Verification items for the finished model (mm, model axes). Face numbers are marked on the shaded views. A direction names the side the tool comes from. Round coordinates to 2 decimals unless told otherwise and drop trailing zeros. Loops run counter-clockwise (first coordinate to the right, second up) from the corner with the lowest first, then second, coordinate; pieces in that order, holes last. Notation, with made-up numbers: M 37,86 L 44,86 A32 cw 44,114 Z; hole C 9.25,-25.5 d10. An arc over 180 degrees is marked long. One line per item, written item: value.
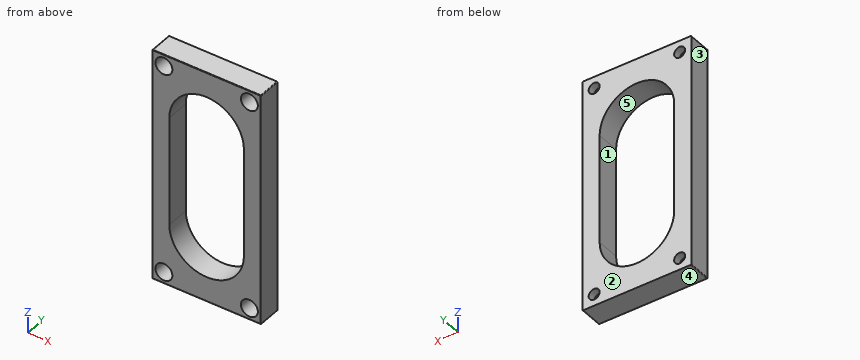
from build123d import *

# Parameters (mm, degrees)
F0_W      = 44.45
F0_H      = 95.25
F0_R      = 3.4671
F1_DEPTH  = 6.35
F0_R_2    = 2.2479
F1_FACE_W = 44.45
F1_FACE_H = 95.25
F1_FACE_R = 3.4671
F2_DEPTH  = 3.175
F3_R      = 0.254


# Not quite as in the source:
# - a feature names something its author has since deleted; it is built from what else it names


with BuildPart() as f1:
    # F0 (on Front) → F1 (new body)
    with BuildSketch(Plane.XZ):
        Rectangle(F0_W, F0_H)
        with Locations((-17.4625, -42.8625)):
            Circle(F0_R, mode=Mode.SUBTRACT)
        with Locations((17.4625, -42.8625)):
            Circle(F0_R, mode=Mode.SUBTRACT)
        with Locations((-17.4625, 42.8625)):
            Circle(F0_R, mode=Mode.SUBTRACT)
        with BuildLine():
            ThreePointArc((-15.24, 22.225), (0, 37.465), (15.24, 22.225))
            Line((15.24, 22.225), (15.24, -22.225))
            ThreePointArc((15.24, -22.225), (0, -37.465), (-15.24, -22.225))
            Line((-15.24, -22.225), (-15.24, 22.225))
        make_face(mode=Mode.SUBTRACT)
        with Locations((17.4625, 42.8625)):
            Circle(F0_R, mode=Mode.SUBTRACT)
    extrude(amount=F1_DEPTH)

    # F0 (on Front) + F1_face (on face) → F2 (join)
    with BuildSketch(Plane.XZ):
        Rectangle(F0_W, F0_H)
        with Locations((-17.4625, -42.8625)):
            Circle(F0_R, mode=Mode.SUBTRACT)
        with Locations((17.4625, -42.8625)):
            Circle(F0_R, mode=Mode.SUBTRACT)
        with Locations((-17.4625, 42.8625)):
            Circle(F0_R, mode=Mode.SUBTRACT)
        with BuildLine():
            ThreePointArc((-15.24, 22.225), (0, 37.465), (15.24, 22.225))
            Line((15.24, 22.225), (15.24, -22.225))
            ThreePointArc((15.24, -22.225), (0, -37.465), (-15.24, -22.225))
            Line((-15.24, -22.225), (-15.24, 22.225))
        make_face(mode=Mode.SUBTRACT)
        with Locations((17.4625, 42.8625)):
            Circle(F0_R, mode=Mode.SUBTRACT)
        with Locations((-17.4625, 42.8625)):
            Circle(F0_R)
        with Locations((-17.4625, 42.8625)):
            Circle(F0_R_2, mode=Mode.SUBTRACT)
        with Locations((17.4625, 42.8625)):
            Circle(F0_R)
        with Locations((17.4625, 42.8625)):
            Circle(F0_R_2, mode=Mode.SUBTRACT)
        with Locations((-17.4625, -42.8625)):
            Circle(F0_R)
        with Locations((-17.4625, -42.8625)):
            Circle(F0_R_2, mode=Mode.SUBTRACT)
        with Locations((17.4625, -42.8625)):
            Circle(F0_R)
        with Locations((17.4625, -42.8625)):
            Circle(F0_R_2, mode=Mode.SUBTRACT)
    with BuildSketch(Plane.XZ.offset(6.35)):
        Rectangle(F1_FACE_W, F1_FACE_H)
        with Locations((-17.4625, -42.8625)):
            Circle(F1_FACE_R, mode=Mode.SUBTRACT)
        with Locations((17.4625, -42.8625)):
            Circle(F1_FACE_R, mode=Mode.SUBTRACT)
        with Locations((-17.4625, 42.8625)):
            Circle(F1_FACE_R, mode=Mode.SUBTRACT)
        with BuildLine():
            Line((-15.24, -22.225), (-15.24, 22.225))
            ThreePointArc((-15.24, 22.225), (0, 37.465), (15.24, 22.225))
            Line((15.24, 22.225), (15.24, -22.225))
            ThreePointArc((15.24, -22.225), (0, -37.465), (-15.24, -22.225))
        make_face(mode=Mode.SUBTRACT)
        with Locations((17.4625, 42.8625)):
            Circle(F1_FACE_R, mode=Mode.SUBTRACT)
    extrude(amount=F2_DEPTH)

    # F3
    f3_edges = [f1.edges().sort_by_distance(p)[0] for p in [
        (-22.225, -9.525, 0),
        (0, -9.525, -47.625),
        (22.225, -9.525, 0),
        (0, -9.525, 47.625),
        (-22.225, -4.7625, 47.625),
        (22.225, -4.7625, 47.625),
        (22.225, -4.7625, -47.625),
        (-22.225, -4.7625, -47.625),
    ]]
    fillet(f3_edges, radius=F3_R)


solid = f1.part
(1) Depth check by flat-ended pin: pin 1 Ø9 at (x, z) = (17.46, -42.86) entering from +Y; pin 2 Ø3.5 at (x, z) = (17, -42) entering from -Y (3 decimals); pin 3 Ø4 at (x, z) = (17.46, -42.86) entering from -Y. Enter the tip coordinate at first touch or a pass-through.
Completed:
pin 1: stops at y = 0
pin 2: stops at y = -3.175
pin 3: passes through
(2) Sectioned sample at C-C on y = -1.75. Count the separate pieces of the cut face and the enclosed holes in it, and give its area (3 significant figures).
Completed:
separate pieces: 1
enclosed holes: 5
area: 2,090 mm^2
(3) Tool access check on the marked faces 1 and 2. Record the directions out of +Z, -Z, +X, -X, +Y, -Y that give a thin tool (end or side, any length) a straight path to the whole face; none if there is none.
Completed:
face 1: +Y, -Y
face 2: +Z, -Z, +X, -X, +Y
(4) Sectioned sample at B-B on z = -9. Enter the section's corners in (x, y) (3 decimals).
Completed:
outline: M -22.225,-9.271 A0.254 ccw -21.971,-9.525 L -15.24,-9.525 L -15.24,0 L -22.225,0 Z; M 15.24,-9.525 L 21.971,-9.525 A0.254 ccw 22.225,-9.271 L 22.225,0 L 15.24,0 Z
(5) Sectioned sample at A-A on x = 0. Enter the section's corners in (y, z) (3 decimals), and give its area (3 significant figures).
Completed:
outline: M -9.525,-47.371 A0.254 ccw -9.271,-47.625 L 0,-47.625 L 0,-37.465 L -9.525,-37.465 Z; M -9.525,37.465 L 0,37.465 L 0,47.625 L -9.271,47.625 A0.254 ccw -9.525,47.371 Z
area: 194 mm^2
(6) Sectioned sample at D-D on z = -42. Enter the section's corners in (x, y) (3 decimals), and give its area (3 significant figures).
Completed:
outline: M -22.225,-9.271 A0.254 ccw -21.971,-9.525 L -20.821,-9.525 L -20.821,-3.175 L -19.538,-3.175 L -19.538,0 L -22.225,0 Z; M -15.387,-3.175 L -14.104,-3.175 L -14.104,-9.525 L 14.104,-9.525 L 14.104,-3.175 L 15.387,-3.175 L 15.387,0 L -15.387,0 Z; M 19.538,-3.175 L 20.821,-3.175 L 20.821,-9.525 L 21.971,-9.525 A0.254 ccw 22.225,-9.271 L 22.225,0 L 19.538,0 Z
area: 312 mm^2
(7) Mould release check, pull along X, two halves, no side actions. Record for the marked faces 3, 4 and 5: +X half, -X half, draft (parallel to the pull), parting line (faces both ways), or undercut.
Completed:
face 3: -X half
face 4: draft
face 5: undercut
(8) Thickness scan on L1, parallel to Z at x = -17.5, y = -1.25 (3 decimals); L2, parallel to X at y = -2.75, z = 18 (3 decimals); L3, parallel to Z at x = -16.5, y = -7.75 (3 decimals). Record the ranges inside material, lowest first. Write a range as from..to.
Completed:
L1: z = -47.625..-45.11, -40.615..40.615, 45.11..47.625
L2: x = -22.225..-15.24, 15.24..22.225
L3: z = -47.625..-46.193, -39.532..39.532, 46.193..47.625
